Here's how the part is built. I have some questions about the finished solid (model axes, mm). Coordinates: 2 decimals unless noted, no trailing zeros. Write each loop counter-clockwise with the first axis right and the second up, starting at its lowest first coordinate (ties: lowest second). Pieces come first, ordered by that corner, then holes. Notation, with made-up numbers: (-30, -30) -> (8, -30) arc R30 ccw to (8, -1) -> close; hole circle Ø7 at (-20.75, 80.25). An arc over 180 degrees is marked (long way). Use a Markdown table: item, result. Add a question column.
Item 1: Imagine slicing it at C-C, the plane y = 7.5. Write out the boundary of the cut face in (x, z) (3 decimals), and give its area (3 significant figures).
Item 2: If we mould it in two halves opening along Y, with no side actions, what happens to faces 1 (the cylindrical face through (9.605, 3.098, 1.999)), 2 (the cylindrical face through (0.14, 9.43, 2)), 3 (the cylindrical face through (0.06, -9.43, 2)), 4 (the cylindrical face through (-5.513, 3.684, 1.282))? For each: pulls with the +Y half, pulls with the -Y half, needs draft (parallel to the pull), parting line crosses it, or undercut.
Item 3: Imagine slicing it at A-A, the plane x = 3.75. Write out the boundary of the cut face in (y, z), and give its area (3 significant figures).
Item 4: Imagine slicing it at B-B, the plane z = 1.35. Write out the boundary of the cut face in (x, y) (3 decimals), and give its area (3 significant figures).
Item 5: Will these pins go through, and if not, where does the flat tip stop? pin 1 Ø2.5 at (x, y) = (6.25, 5.01) entering from -Z; pin 2 Ø3 at (x, y) = (-2, 0) entering from -Z; pin 3 Ø1.5 at (y, z) = (-7, 0.5) entering from +X.
Item 6: Imagine slicing it at D-D, the plane z = 0.25. Write out the boundary of the cut face in (x, y) (3 decimals).
Item 7: If I drill on line 1 along X through (y, z) = (4.25, 0.5) (3 decimals); line 2 along X through (y, z) = (0.5, 1.65); line 3 along Y through (x, z) = (6, 0.45), over which ranges is the centre line in solid material (lowest first)? Write a range as from..to.
```python
from build123d import *

# Parameters (mm, degrees)
F0_W     = 20.35
F0_H     = 20
F1_DEPTH = 2.6
F2_R     = 1.5
F3_DEPTH = 25
F4_R     = 0.95
F5_DEPTH = 25
F6_R     = 6
F7_R     = 2


with BuildPart() as f1:
    # F0 (on Top) → F1 (new body)
    with BuildSketch(Plane.XY):
        Rectangle(F0_W, F0_H)
    extrude(amount=F1_DEPTH)

    # F2 (on Top) → F3 (cut)
    with BuildSketch(Plane.XY):
        with Locations((-6.2053604051, 5.0143129192)):
            Circle(F2_R)
        with Locations((6.2522287481, 5.0141313113)):
            Circle(F2_R)
    extrude(amount=F3_DEPTH, mode=Mode.SUBTRACT)

    # F4 (on Top) → F5 (cut)
    with BuildSketch(Plane.XY):
        with Locations((-4.2495448142, 0.3267968714)):
            Circle(F4_R)
        with Locations((4.2728632689, 0.318708655)):
            Circle(F4_R)
    extrude(amount=F5_DEPTH, mode=Mode.SUBTRACT)

    # F6
    f6_edges = [f1.edges().sort_by_distance(p)[0] for p in [
        (10.175, -10, 1.3),
        (-10.175, -10, 1.3),
    ]]
    fillet(f6_edges, radius=F6_R)

    # F7
    f7_edges = [f1.edges().sort_by_distance(p)[0] for p in [
        (-8.417641, -8.242641, 2.6),
        (8.417641, -8.242641, 2.6),
        (10.175, 3, 2.6),
        (0, 10, 2.6),
        (-10.175, 3, 2.6),
        (0, -10, 2.6),
    ]]
    fillet(f7_edges, radius=F7_R)


solid = f1.part
```
Ans:
| question | item | result |
|---|---|---|
| 1 | outline | (-10.175, 0) -> (10.175, 0) -> (10.175, 0.6) arc R2 ccw to (8.175, 2.6) -> (-8.175, 2.6) arc R2 ccw to (-10.175, 0.6) -> close |
| 1 | area | 51.2 mm^2 |
| 2 | face 1 | needs draft |
| 2 | face 2 | pulls with the +Y half |
| 2 | face 3 | pulls with the -Y half |
| 2 | face 4 | undercut |
| 3 | outline | (-10, 0) -> (-0.47, 0) -> (-0.47, 2.6) -> (-8, 2.6) arc R2 ccw to (-10, 0.6) -> close; (1.11, 0) -> (10, 0) -> (10, 0.6) arc R2 ccw to (8, 2.6) -> (1.11, 2.6) -> close |
| 3 | area | 46.2 mm^2 |
| 4 | outline | (-10.029, -4) arc R5.854 ccw to (-4.175, -9.854) -> (4.175, -9.854) arc R5.854 ccw to (10.029, -4) -> (10.029, 9.854) -> (-10.029, 9.854) -> close; hole circle Ø3 at (-6.205, 5.014); hole circle Ø1.9 at (-4.25, 0.327); hole circle Ø1.9 at (4.273, 0.319); hole circle Ø3 at (6.252, 5.014) |
| 4 | area | 361 mm^2 |
| 5 | pin 1 | passes through |
| 5 | pin 2 | stops at z = 0 |
| 5 | pin 3 | stops at x = 9.74 |
| 6 | outline | (-10.175, -4) arc R6 ccw to (-4.175, -10) -> (4.175, -10) arc R6 ccw to (10.175, -4) -> (10.175, 10) -> (-10.175, 10) -> close; hole circle Ø3 at (-6.205, 5.014); hole circle Ø1.9 at (-4.25, 0.327); hole circle Ø1.9 at (4.273, 0.319); hole circle Ø3 at (6.252, 5.014) |
| 7 | line 1 | x = -10.175..-7.496, -4.915..4.961, 7.543..10.175 |
| 7 | line 2 | x = -9.88..-5.18, -3.32..3.34, 5.21..9.88 |
| 7 | line 3 | y = -9.72..3.54, 6.49..10 |
